Verification items for this drawing (mm, ordinates from the low corner). Round coordinates to 2 decimals unless told otherwise and drop trailing zeros. Order: outer loops, then holes, each group sorted by start corner. A loop starts at its lowest first (then second) coordinate and runs counter-clockwise, first axis right, second up. Notation, with made-up numbers: (83, -25) - (97, -25) arc R27 ccw to (97, 4) - close; hole circle Ø1 at (-12.5, 23). An arc over 180 degrees is marked (long way). Use a Markdown table: item, result. Add a question column.
(1) Mould release check, pull along X, two halves, no side actions. Record for the marked faces 1, 2 and 3: released by +X, released by -X, zero draft, split by the parting line, or undercut.
(2) Thickness scan on line 1 along Y through (x, z) = (20, 3.45); line 2 along X through (y, z) = (25.5, 2.75); line 3 along X through (y, z) = (16, 3.5). Record the ranges inside material, lowest first. Write a range as [from, to].
(3) Section check B-B on y = 20. Record the boundary of the cut face in (x, z).
(4) Section check A-A on z = 1.5. Record the boundary of the cut face in (x, y), then the cut area to 3 significant figures.
(5) Section check D-D on y = 4. Record the boundary of the cut face in (x, z).
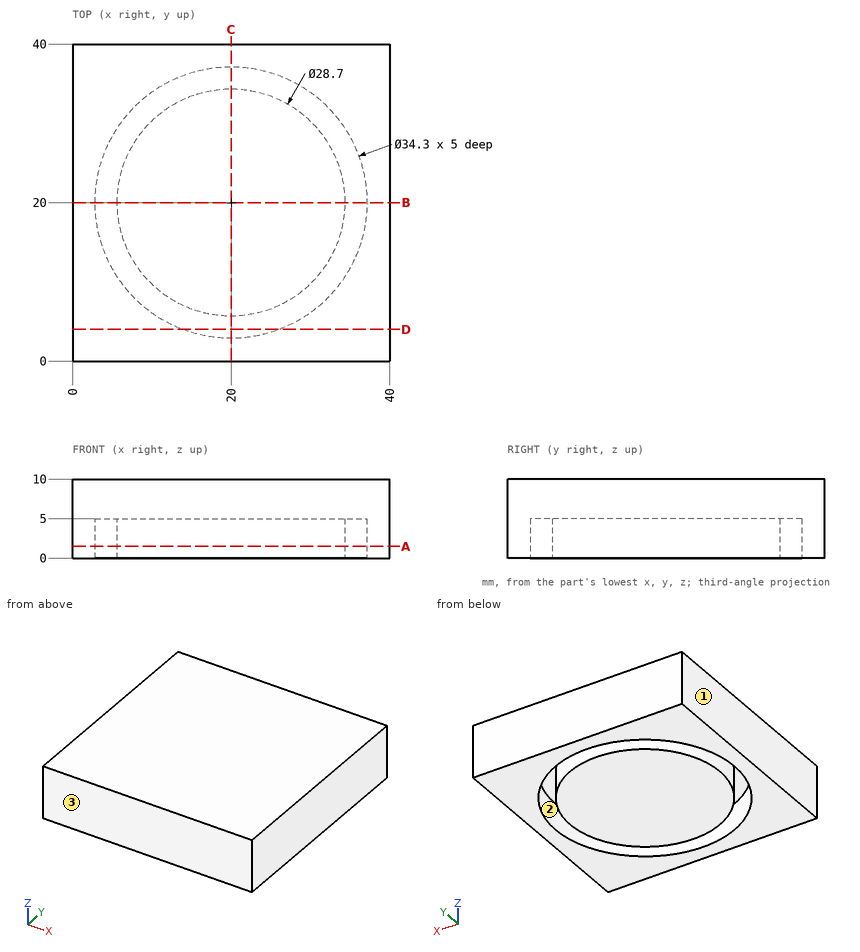
Check sheet entries:
| question | item | result |
|---|---|---|
| 1 | face 1 | released by -X |
| 1 | face 2 | undercut |
| 1 | face 3 | zero draft |
| 2 | line 1 | y = [0, 2.85], [5.65, 34.35], [37.15, 40] |
| 2 | line 2 | x = [0, 3.76], [6.75, 33.25], [36.24, 40] |
| 2 | line 3 | x = [0, 3.32], [6.22, 33.78], [36.68, 40] |
| 3 | outline | (0, 0) - (2.85, 0) - (2.85, 5) - (5.65, 5) - (5.65, 0) - (34.35, 0) - (34.35, 5) - (37.15, 5) - (37.15, 0) - (40, 0) - (40, 10) - (0, 10) - close |
| 4 | outline | (0, 0) - (40, 0) - (40, 40) - (0, 40) - close; circle Ø28.7 at (20, 20); hole circle Ø34.3 at (20, 20) |
| 4 | area | 1,320 mm2 |
| 5 | outline | (0, 0) - (13.83, 0) - (13.83, 5) - (26.17, 5) - (26.17, 0) - (40, 0) - (40, 10) - (0, 10) - close |
